Work out the finished part from the listing and answer in its coordinate system (mm). A direction names the side the tool comes from. Give positions to 0.01 mm unless a question says otherwise; leave off trailing zeros. Order: outer loops, then holes, each group sorted by start corner. A loop starts at its lowest first (then second) coordinate and runs counter-clockwise, first axis right, second up.
```python
from build123d import *

# Parameters (mm, degrees)
SKETCH125_W     = 56.5
SKETCH125_H     = 22
PAD023_DEPTH    = 25
SKETCH126_W     = 40.5
SKETCH126_H     = 19
POCKET095_DEPTH = 20
POCKET096_DEPTH = 25
SKETCH128_W     = 3
SKETCH128_H     = 5.8
POCKET098_DEPTH = 56.5
SKETCH130_R     = 1.6
POCKET099_DEPTH = 8.5
POCKET100_DEPTH = 8
FILLET035_R     = 0.5
SKETCH132_R     = 0.95
POCKET101_DEPTH = 3
POCKET102_DEPTH = 1.5
FILLET036_R     = 5
FILLET037_R     = 1
SKETCH_W        = 56.5
SKETCH_H        = 5
PAD_DEPTH       = 10
FILLET_R        = 0.4


with BuildPart() as part:
    # Sketch125 → Pad023 (new body)
    with BuildSketch(Plane.XY):
        with Locations((28.25, -11)):
            Rectangle(SKETCH125_W, SKETCH125_H)
    extrude(amount=PAD023_DEPTH)

    # Sketch126 (on Face6 of Pad023) → Pocket095 (cut)
    with BuildSketch(Plane.XY.offset(25)):
        with Locations((28.25, -9.5)):
            Rectangle(SKETCH126_W, SKETCH126_H)
    extrude(amount=-POCKET095_DEPTH, mode=Mode.SUBTRACT)

    # Sketch127 (on Face4 of Pocket095) → Pocket096 (cut)
    with BuildSketch(Plane.XY.offset(25)):
        with BuildLine():
            ThreePointArc((0, -16), (10.856869, -20.474241), (22.5, -22))
            Line((22.5, -22), (56.5, -22))
            Line((56.5, -22), (56.5, -23))
            Line((56.5, -23), (0, -23))
            Line((0, -23), (0, -16))
        make_face()
    extrude(amount=-POCKET096_DEPTH, mode=Mode.SUBTRACT)

    # Sketch128 (on Face3 of Pocket096) → Pocket098 (cut)
    with BuildSketch(Plane.YZ.offset(56.5)):
        with Locations((-4.5, 20)):
            Rectangle(SKETCH128_W, SKETCH128_H)
        with Locations((-4.5, 10)):
            Rectangle(SKETCH128_W, SKETCH128_H)
    extrude(amount=-POCKET098_DEPTH, mode=Mode.SUBTRACT)

    # Sketch130 (on Face1 of Pocket098) → Pocket099 (cut)
    with BuildSketch(Plane(origin=(0, 0, 0), x_dir=(-1, 0, 0), z_dir=(0, 1, 0))):
        with Locations((-52.5, 20)):
            Circle(SKETCH130_R)
        with Locations((-52.5, 10)):
            Circle(SKETCH130_R)
        with Locations((-4, 20)):
            Circle(SKETCH130_R)
        with Locations((-4, 10)):
            Circle(SKETCH130_R)
    extrude(amount=-POCKET099_DEPTH, mode=Mode.SUBTRACT)

    # Sketch131 (on Face4 of Pocket099) → Pocket100 (cut)
    with BuildSketch(Plane.YZ.offset(56.5)):
        with BuildLine():
            ThreePointArc((-14.5, 11.5), (-12, 9), (-9.5, 11.5))
            Line((-9.5, 25), (-9.5, 11.5))
            Line((-14.5, 25), (-9.5, 25))
            Line((-14.5, 11.5), (-14.5, 25))
        make_face()
    extrude(amount=-POCKET100_DEPTH, mode=Mode.SUBTRACT)

    # Fillet035
    fillet035_edges = [part.edges().sort_by_distance(p)[0] for p in [
        (52.5, -9.5, 25),
        (52.5, -14.5, 25),
    ]]
    fillet(fillet035_edges, radius=FILLET035_R)

    # Sketch132 (on Face4 of Fillet035) → Pocket101 (cut)
    with BuildSketch(Plane.XZ.offset(22)):
        with Locations((38.25, 15)):
            Circle(SKETCH132_R)
    extrude(amount=-POCKET101_DEPTH, mode=Mode.SUBTRACT)

    # Sketch133 (on Face22 of Pocket101) → Pocket102 (cut)
    with BuildSketch(Plane(origin=(0, -19, 0), x_dir=(-1, 0, 0), z_dir=(0, 1, 0))):
        Polygon((-36.2, 16.183568), (-38.25, 17.367136), (-40.3, 16.183568), (-40.3, 13.816432), (-38.25, 12.632864), (-36.2, 13.816432), align=None)
    extrude(amount=-POCKET102_DEPTH, mode=Mode.SUBTRACT)

    # Fillet036
    fillet036_edges = [part.edges().sort_by_distance(p)[0] for p in [
        (56.5, -22, 12.5),
    ]]
    fillet(fillet036_edges, radius=FILLET036_R)

    # Fillet037
    fillet037_edges = [part.edges().sort_by_distance(p)[0] for p in [
        (8, -19, 15),
        (48.5, -19, 15),
        (48.5, -9.5, 5),
        (28.25, -19, 5),
        (8, -9.5, 5),
    ]]
    fillet(fillet037_edges, radius=FILLET037_R)

    # Sketch (on Face11 of Fillet037) → Pad (join)
    with BuildSketch(Plane(origin=(0, 0, 0), x_dir=(-1, 0, 0), z_dir=(0, 1, 0))):
        with Locations((-28.25, 2.5)):
            Rectangle(SKETCH_W, SKETCH_H)
    extrude(amount=PAD_DEPTH)

    # Fillet
    fillet_edges = [part.edges().sort_by_distance(p)[0] for p in [
        (56.5, 10, 2.5),
        (0, 10, 2.5),
    ]]
    fillet(fillet_edges, radius=FILLET_R)


solid = part.part
```
1. The part is cut by section C-C (z = 20). State how many separate pieces and enclosed holes the cut face has, then the cut area to 3 significant figures.
Findings below:
separate pieces: 6
enclosed holes: 0
area: 302 mm2
2. Straight lines are drawn through the part: probe 1 along Z at (x, y) = (52.5, -7); probe 2 along X at (y, z) = (-7, 6.25); probe 3 along Y at (x, z) = (47, 10.25). For each, find the intervals that lie inside material, in ascending order.
Findings below:
probe 1: z = 0 to 8.4, 11.6 to 18.4, 21.6 to 25
probe 2: x = 0 to 8, 48.5 to 56.5
probe 3: y = -22 to -19
3. Given P1, Ø1.5, axis at x = 9, z = 13, coming from the -Y side; P2, Ø2, axis at x = 21.5, y = 4, coming from the -Z side; P3, Ø4.5, axis at x = 54, z = 13, coming from the +Y side; P4, Ø1.9, axis at x = 4, z = 10, coming from the +Y side, each flat-ended and moving along its own axis, determine where each tip first touches the part or whether it passes through.
Findings below:
P1: stops at y = -20.16
P2: stops at z = 0
P3: stops at y = 0
P4: stops at y = -8.5
4. Which of the six approach directions +Z, -Z, +X, -X, +Y, -Y give full straight-line access (tool end or side, diameter ignored) to faces 5 (the face through (4.208, -1.479, 21.586)), 6 (the face through (4, -5, 12.9)), 7 (the face through (53, -14.5, 18)), 8 (the face through (29, -4, 5))?
Findings below:
face 5: +Y
face 6: +X, -X
face 7: +Z, +X
face 8: +Z, +Y
5. The part is cut by section A-A (y = -7.5). Write down the section's boundary in (x, z).
Findings below:
outline: (0, 0) - (56.5, 0) - (56.5, 25) - (48.5, 25) - (48.5, 6) arc R1 cw to (47.5, 5) - (9, 5) arc R1 cw to (8, 6) - (8, 25) - (0, 25) - close; hole circle Ø3.2 at (4, 10); hole circle Ø3.2 at (4, 20); hole circle Ø3.2 at (52.5, 10); hole circle Ø3.2 at (52.5, 20)
6. The part is cut by section D-D (y = -12). Write down the section's boundary in (x, z), then the cut area to 3 significant figures.
Findings below:
outline: (0, 0) - (56.5, 0) - (56.5, 9) - (48.5, 9) - (48.5, 6) arc R1 cw to (47.5, 5) - (9, 5) arc R1 cw to (8, 6) - (8, 25) - (0, 25) - close
area: 475 mm2
7. The mould has two halves that part along Y. Classify faces 1 (the face through (52, -4, 25)), 2 (the face through (53, -5, 22.9)), 3 (the face through (29, 10, 3)), 4 (the face through (4, -5, 22.9)): pulls with the +Y half, pulls with the -Y half, needs draft (parallel to the pull), parting line crosses it, or undercut.
Findings below:
face 1: needs draft
face 2: undercut
face 3: pulls with the +Y half
face 4: undercut
